from build123d import *

# Parameters (mm, degrees)
F0_W     = 48
F0_H     = 48
F1_DEPTH = 800
F2_W     = 30
F2_H     = 30
F3_DEPTH = 50
F4_W     = 30
F4_H     = 30
F5_DEPTH = 50


with BuildPart() as f1:
    # F0 (on Front) → F1 (new body)
    with BuildSketch(Plane.XZ):
        Rectangle(F0_W, F0_H)
    extrude(amount=-F1_DEPTH)

    # F2 (on face) → F3 (join)
    with BuildSketch(Plane.XY.offset(24)):
        with Locations((0, 423)):
            Rectangle(F2_W, F2_H)
    extrude(amount=F3_DEPTH)

    # F4 (on face) → F5 (join)
    with BuildSketch(Plane(origin=(0, 0, -24), x_dir=(1, 0, 0), z_dir=(0, 0, -1))):
        with Locations((0, -423)):
            Rectangle(F4_W, F4_H)
    extrude(amount=F5_DEPTH)


solid = f1.part
Build history of the part. All positions in model axes, mm. A direction names the side the tool comes from. Give positions to 0.01 mm unless a question says otherwise; leave off trailing zeros. Order: outer loops, then holes, each group sorted by start corner. A loop starts at its lowest first (then second) coordinate and runs counter-clockwise, first axis right, second up. Notation, with made-up numbers: M 57.5,34.5 L 86.5,34.5 A24 ccw 86.5,64.5 Z; hole C 34.25,2.5 d6. An arc over 180 degrees is marked long. Put each result on its own line as item: value.
Item 1: Flat gauge pins, fed straight in: pin 1 Ø9 at (y, z) = (416.5, 43.5) entering from -X; pin 2 Ø24 at (y, z) = (418.5, 43.5) entering from +X; pin 3 Ø5 at (x, y) = (9.5, 157) entering from +Z; pin 4 Ø8 at (x, z) = (-10.5, 7) entering from -Y. Where does each tip first touch, or does it go through?
From the geometry:
pin 1: stops at x = -15
pin 2: stops at x = 15
pin 3: stops at z = 24
pin 4: stops at y = 0
Item 2: 3-axis set-ups, long thin cutter, end or side, ignore diameter. For faces 1 (the flat face through (0, 408, -49)), 2 (the flat face through (0, 438, 49)), 3 (the flat face through (15, 423, -49)), 4 (the flat face through (-15, 423, -49)), 5 (the flat face through (15, 423, 49)): which of +Z, -Z, +X, -X, +Y, -Y reach the whole face in a straight line?
From the geometry:
face 1: -Z, +X, -X, -Y
face 2: +Z, +X, -X, +Y
face 3: -Z, +X, +Y, -Y
face 4: -Z, -X, +Y, -Y
face 5: +Z, +X, +Y, -Y
Item 3: Slice it at C-C, the plane y = 505. Write the cut outline in (x, z).
From the geometry:
outline: M -24,-24 L 24,-24 L 24,24 L -24,24 Z
Item 4: Slice it at B-B, the plane z = -63.5. Write the cut outline in (x, y).
From the geometry:
outline: M -15,408 L 15,408 L 15,438 L -15,438 Z
Item 5: Slice it at A-A, the plane x = -3. Write the cut outline in (y, z), plus the area to 3 significant figures.
From the geometry:
outline: M 0,-24 L 408,-24 L 408,-74 L 438,-74 L 438,-24 L 800,-24 L 800,24 L 438,24 L 438,74 L 408,74 L 408,24 L 0,24 Z
area: 41,400 mm2
Item 6: Probe line 1 (Z direction, x = 6, y = 466); line 2 (Y direction, x = 14.5, z = 56). List the from-to ranges inside material, lowest first. Write a range as [from, to].
From the geometry:
line 1: z = [-24, 24]
line 2: y = [408, 438]
